For this review, take the finished solid that the model builds, in its own axes (mm). Face numbers are marked on the shaded views. A direction names the side the tool comes from. Coordinates: 2 decimals unless noted, no trailing zeros. Write each loop counter-clockwise with the first axis right and the second up, starting at its lowest first coordinate (ties: lowest second). Pieces come first, ordered by that corner, then holes. Notation, with made-up numbers: (-38, -13.75) -> (12, -13.75) arc R20 ccw to (12, 0.25) -> close; hole circle Ø11 at (9.25, 16). An arc over 180 degrees is marked (long way). One line per item, written item: value. Start each with the question number.
1) For probe 1 along Z at (x, y) = (14.5, 1.5); probe 2 along X at (y, z) = (5, 0.5); probe 3 along X at (y, z) = (-2, -4.25), list the stretches that pass through material, from the lowest coordinate up. Write a range as from..to.
2) Mouldability with a two-part tool opening along X and no side actions: class the marked faces 3, 4 and 5 as released by +X, released by -X, zero draft, split by the parting line, or undercut.
3) Add section C-C (y = -5.75). State the section outline as (x, z) points, and give its area (3 significant figures).
4) For pin 1 Ø3 at (x, z) = (81, 0.5) entering from -Y; pin 2 Ø4 at (x, y) = (48, 7) entering from +Z; pin 3 Ø0.5 at (x, z) = (16.5, -3) entering from +Y, all flat-tipped, find the tip position at first contact; note any pin that passes through.
5) Add section A-A (y = 3). State the section outline as (x, z) points, and give its area (3 significant figures).
6) Add section B-B (z = 1.25). State the section outline as (x, y) points, and give its area (3 significant figures).
7) Machinability: for the marked faces 1 and 2, which of the approach directions +Z, -Z, +X, -X, +Y, -Y give a long, thin tool a straight path to every point of the face, cutting with its end or side? Answer none if there is none.
from build123d import *

# Parameters (mm, degrees)
BLANKSKE_W         = 100
BLANKSKE_H         = 11.5
BLANK_DEPTH        = 5
TOOTHCUTSIM_DEPTH  = 101.783183121
TEETHCUTS_COUNT    = 22
TEETHCUTS_PITCH    = 4.712388975
BOSS_EXTRU_1_DEPTH = 5
BOSS_EXTRU_2_DEPTH = 5


with BuildPart() as part:
    # BlankSke → Blank (new body)
    with BuildSketch(Plane.XY):
        with Locations((50, 5.75)):
            Rectangle(BLANKSKE_W, BLANKSKE_H)
    extrude(amount=-BLANK_DEPTH)

    # TooCutSkeSim → ToothCutSim (cut, through all)
    with BuildSketch(Plane.XY):
        Polygon((0.654653055, 8.125), (-0.654653055, 8.125), (-1.892297439, 11.5254), (1.892297439, 11.5254), align=None)
    toothcutsim = extrude(amount=-TOOTHCUTSIM_DEPTH, mode=Mode.SUBTRACT)

    # TeethCuts: ToothCutSim ×22
    with Locations(*[(i * TEETHCUTS_PITCH, 0, 0) for i in range(1, TEETHCUTS_COUNT)]):
        add(toothcutsim, mode=Mode.SUBTRACT)

    # Esquisse1 → Boss.-Extru.1 (add)
    with BuildSketch(Plane(origin=(100, 0, 0), x_dir=(0, 0, -1), z_dir=(1, 0, 0))):
        with BuildLine():
            Line((5, 12.18326915), (0, 12.18326915))
            ThreePointArc((0, 12.18326915), (-2.121320344, 11.304589494), (-3, 9.18326915))
            Line((-3, 9.18326915), (-3, 0))
            ThreePointArc((-3, 0), (-2.121320344, -2.121320344), (0, -3))
            Line((0, -3), (5, -3))
            ThreePointArc((5, -3), (7.121320344, -2.121320344), (8, 0))
            Line((8, 0), (8, 9.18326915))
            ThreePointArc((8, 9.18326915), (7.121320344, 11.304589494), (5, 12.18326915))
        make_face()
    extrude(amount=BOSS_EXTRU_1_DEPTH)

    # Esquisse2 → Boss.-Extru.2 (add)
    with BuildSketch(Plane(origin=(0, 0, -5), x_dir=(-1, 0, 0), z_dir=(0, 0, -1))):
        with BuildLine():
            Line((0, 8.125), (0.072259216, 8.125))
            ThreePointArc((0.072259216, 8.125), (0.372641653, 8.225287114), (0.552526139, 8.485918434))
            ThreePointArc((0.552526139, 8.485918434), (5.589291766, 15.783595396), (14, 18.591634575))
            ThreePointArc((14, 18.591634575), (15.25, 17.341634575), (14, 16.091634575))
            ThreePointArc((14, 16.091634575), (2.5, 4.591634575), (14, -6.908365425))
            ThreePointArc((14, -6.908365425), (15.25, -8.158365425), (14, -9.408365425))
            ThreePointArc((14, -9.408365425), (6.025818336, -6.915425292), (0.891516314, -0.324426394))
            ThreePointArc((0.891516314, -0.324426394), (0.708148385, -0.089033576), (0.423356182, 0))
            Line((0.423356182, 0), (0, 0))
            Line((0, 0), (0, 8.125))
        make_face()
    extrude(amount=-BOSS_EXTRU_2_DEPTH)


solid = part.part
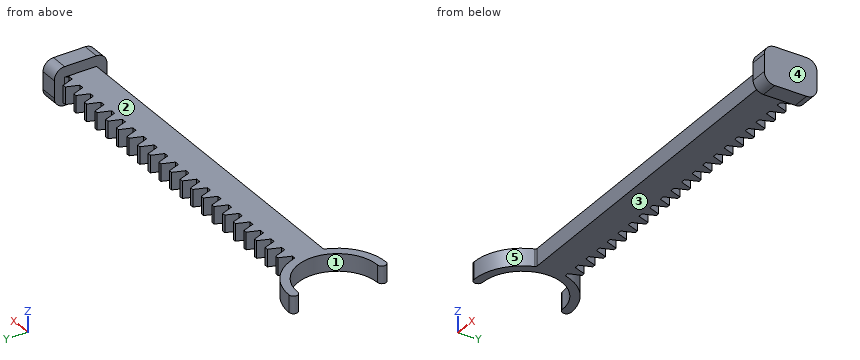
Numbers:
1. probe 1: -5..0
1. probe 2: 100..105
1. probe 3: -4.58..-1.65, 100..105
2. face 3: zero draft
2. face 4: released by +X
2. face 5: undercut
3. outline: (-8.97, -5) -> (-4.56, -5) -> (-4.56, 0) -> (-8.97, 0) -> close
3. area: 22.0 mm²
4. pin 1: y = 0
4. pin 2: z = 0
4. pin 3: y = 11.5
5. outline: (-2.61, -5) -> (100, -5) -> (100, -8) -> (105, -8) -> (105, 3) -> (100, 3) -> (100, 0) -> (-2.61, 0) -> close
5. area: 568 mm²
6. outline: (100, -2.73) -> (105, -2.73) -> (105, 11.91) -> (100, 11.91) -> close
6. area: 73.2 mm²
7. face 1: +Z, -Z, -X
7. face 2: +Z, -X, +Y, -Y
